For this review, take the finished solid that the model builds, in its own axes (mm). Face numbers are marked on the shaded views. A direction names the side the tool comes from. Round coordinates to 2 decimals unless told otherwise and drop trailing zeros. Loops run counter-clockwise (first coordinate to the right, second up) from the corner with the lowest first, then second, coordinate; pieces in that order, holes last.
```python
from build123d import *

# Parameters (mm, degrees)
SKETCH_1_R          = 18.5
EXTRUDE_1_DEPTH     = 22
SKETCH_2_R          = 6
EXTRUDE_2_DEPTH     = 6
SKETCH_3_R          = 3
EXTRUDE_3_DEPTH     = 15.5
CUT_EXTRUDE_1_DEPTH = 12
SKETCH_5_R          = 1.5
CUT_EXTRUDE_2_DEPTH = 6
SKETCH_6_R          = 16.5
EXTRUDE_4_DEPTH     = 22.7
SKETCH_7_R          = 8
EXTRUDE_5_DEPTH     = 6


with BuildPart() as part:
    # 草图1 → 凸台-拉伸1 (new body)
    with BuildSketch(Plane.XY):
        Circle(SKETCH_1_R)
    extrude(amount=EXTRUDE_1_DEPTH)

    # 草图2 → 凸台-拉伸2 (add)
    with BuildSketch(Plane.XY.offset(22)):
        with Locations((0, 7)):
            Circle(SKETCH_2_R)
    extrude(amount=EXTRUDE_2_DEPTH)

    # 草图3 → 凸台-拉伸3 (add)
    with BuildSketch(Plane.XY.offset(28)):
        with Locations((0, 7)):
            Circle(SKETCH_3_R)
    extrude(amount=EXTRUDE_3_DEPTH)

    # 草图4 → 切除-拉伸1 (cut)
    with BuildSketch(Plane.XY.offset(43.5)):
        Polygon((-3.340950009, 9.5), (3.684231377, 9.5), (0.516334163, 11.681498446), align=None)
    extrude(amount=-CUT_EXTRUDE_1_DEPTH, mode=Mode.SUBTRACT)

    # 草图5 → 切除-拉伸2 (cut)
    with BuildSketch(Plane.XY.offset(22)):
        with Locations((15.5, 0)):
            Circle(SKETCH_5_R)
        with Locations((7.75, -13.423393759)):
            Circle(SKETCH_5_R)
        with Locations((-7.75, -13.423393759)):
            Circle(SKETCH_5_R)
        with Locations((-15.5, 0)):
            Circle(SKETCH_5_R)
        with Locations((-7.75, 13.423393759)):
            Circle(SKETCH_5_R)
        with Locations((7.75, 13.423393759)):
            Circle(SKETCH_5_R)
    extrude(amount=-CUT_EXTRUDE_2_DEPTH, mode=Mode.SUBTRACT)

    # 草图6 → 凸台-拉伸4 (add)
    with BuildSketch(Plane(origin=(0, 0, 0), x_dir=(-1, 0, 0), z_dir=(0, 0, -1))):
        with Locations(Location((0, 0, 0), (0, 0, 180))):
            Circle(SKETCH_6_R)
    extrude(amount=EXTRUDE_4_DEPTH)

    # 草图7 → 凸台-拉伸5 (add)
    with BuildSketch(Plane(origin=(0, 0, -22.7), x_dir=(-1, 0, 0), z_dir=(0, 0, -1))):
        Circle(SKETCH_7_R)
    extrude(amount=EXTRUDE_5_DEPTH)


solid = part.part
```
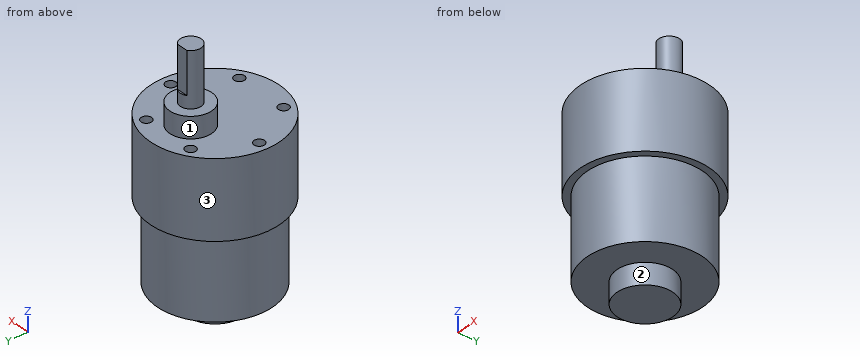
(1) Insertion check: pin 1 Ø3.5 at (x, y) = (7.75, -13.42) entering from -Z; pin 2 Ø1 at (x, z) = (0, 37.5) entering from +Y; pin 3 Ø6 at (x, z) = (-7.5, 12) entering from +Y. Each pin has a flat end and moves straight along its axis. Give the tip position at first contact, or say it passes through.
(2) Add section C-C (z = -2.5). Give the boundary of the cut face in (x, y).
(3) For the marked faces 1, 2 and 3, list the 3-axis set-ups (+Z, -Z, +X, -X, +Y, -Y) from which the entire face can be reached by the end or side of a thin tool; tool diameter is ignored.
(4) For L1, parallel to Y at x = -7.75, z = 17.2; L2, parallel to Z at x = 3.5, y = -16; L3, parallel to Z at x = -5, y = 5, list the stretches that pass through material, from the lowest coordinate up.
(5) Add section A-A (y = 0). Give the boundary of the cut face in (x, z).
(6) Add section D-D (y = -4). Give the boundary of the cut face in (x, z).
(7) Add section B-B (x = 0). Give the boundary of the cut face in (y, z), plus the area to 3 significant figures.
Outcome:
1. pin 1: stops at z = -22.7
1. pin 2: stops at y = 9.5
1. pin 3: stops at y = 17.94
2. outline: circle Ø33 at (0, 0)
3. face 1: +Z
3. face 2: -Z
3. face 3: +Z, -Z
4. L1: y = -16.8 to -14.92, -11.92 to 11.92, 14.92 to 16.8
4. L2: z = -22.7 to 22
4. L3: z = -28.7 to 28
5. outline: (-18.5, 0) - (-16.5, 0) - (-16.5, -22.7) - (-8, -22.7) - (-8, -28.7) - (8, -28.7) - (8, -22.7) - (16.5, -22.7) - (16.5, 0) - (18.5, 0) - (18.5, 22) - (17, 22) - (17, 16) - (14, 16) - (14, 22) - (-14, 22) - (-14, 16) - (-17, 16) - (-17, 22) - (-18.5, 22) - close
6. outline: (-18.06, 0) - (-16.01, 0) - (-16.01, -22.7) - (-6.93, -22.7) - (-6.93, -28.7) - (6.93, -28.7) - (6.93, -22.7) - (16.01, -22.7) - (16.01, 0) - (18.06, 0) - (18.06, 22) - (-18.06, 22) - close
7. outline: (-18.5, 0) - (-16.5, 0) - (-16.5, -22.7) - (-8, -22.7) - (-8, -28.7) - (8, -28.7) - (8, -22.7) - (16.5, -22.7) - (16.5, 0) - (18.5, 0) - (18.5, 22) - (13, 22) - (13, 28) - (10, 28) - (10, 31.5) - (9.5, 31.5) - (9.5, 43.5) - (4, 43.5) - (4, 28) - (1, 28) - (1, 22) - (-18.5, 22) - close
7. area: 1,820 mm2
